```python
from build123d import *

# Parameters (mm, degrees)
SKETCH4_W                = 12.46
SKETCH4_H                = 17.25
BOSS_EXTRUDE3_DEPTH      = 6
SKETCH8_R                = 12.546781182
SKETCH8_R_2              = 11.15
BOSS_EXTRUDE6_DEPTH      = 8.3
BOSS_EXTRUDE6_DEPTH_BACK = 17.25
BOSS_EXTRUDE4_DEPTH      = 17.25
SKETCH6_R                = 0.75
CUT_EXTRUDE1_DEPTH       = 5
CHAMFER1_SIZE            = 0.5
CHAMFER1_SIZE2           = 0.866025404
SKETCH10_W               = 12.46
SKETCH10_H               = 23.7
CUT_EXTRUDE3_DEPTH       = 17.25
BOSS_EXTRUDE7_DEPTH      = 8.3
BOSS_EXTRUDE9_DEPTH      = 10
SKETCH20_R               = 11.15
SKETCH20_R_2             = 7.15
BOSS_EXTRUDE11_DEPTH     = 8.3
SKETCH21_R               = 10.15
SKETCH21_R_2             = 7.15
CUT_EXTRUDE7_DEPTH       = 1.3
SKETCH11_W               = 10
SKETCH11_H               = 2
CUT_EXTRUDE4_DEPTH       = 23.7
CUT_EXTRUDE8_REACH       = 37.55
SKETCH25_W               = 12.46
SKETCH25_H               = 6
BOSS_EXTRUDE10_DEPTH     = 35.55
SKETCH18_W               = 21.5
SKETCH18_H               = 11.438292938
CUT_EXTRUDE5_DEPTH       = 2
SKETCH19_R               = 3.5
CUT_EXTRUDE6_DEPTH       = 43.5
CUT_EXTRUDE6_DEPTH_BACK  = 3
FILLET1_R                = 10
SKETCH22_R               = 6.5
BOSS_EXTRUDE12_DEPTH     = 5
SKETCH23_R               = 6.075
BOSS_EXTRUDE13_DEPTH     = 5
FILLET2_R                = 1
BOSS_EXTRUDE14_DEPTH     = 2
CUT_EXTRUDE9_REACH       = 46.5
SKETCH27_R               = 0.75


with BuildPart() as part:
    # Sketch4 → Boss-Extrude3 (new body)
    with BuildSketch(Plane.XY):
        with Locations((0, -1.35)):
            Rectangle(SKETCH4_W, SKETCH4_H)
    extrude(amount=BOSS_EXTRUDE3_DEPTH)



with BuildPart() as body_2:
    # Sketch8 → Boss-Extrude6 (new body, two sides)
    with BuildSketch(Plane(origin=(0, -9.975, 0), x_dir=(-1, 0, 0), z_dir=(0, -1, 0))) as boss_extrude6_sk:
        with Locations((0, -23.55)):
            Circle(SKETCH8_R)
        with Locations((0, -23.55)):
            Circle(SKETCH8_R_2, mode=Mode.SUBTRACT)
    extrude(amount=BOSS_EXTRUDE6_DEPTH)
    extrude(boss_extrude6_sk.sketch, amount=-BOSS_EXTRUDE6_DEPTH_BACK)


with BuildPart() as part_1:
    add(part.part)

    add(body_2.part)  # Boss-Extrude4 merges body 2
    # Sketch5 → Boss-Extrude4 (add)
    with BuildSketch(Plane(origin=(0, 7.275, 0), x_dir=(1, 0, 0), z_dir=(0, 1, 0))):
        with BuildLine():
            Line((12.546781182, -23.55), (12.546781182, 0))
            Line((12.546781182, 0), (6.23, 0))
            Line((6.23, 0), (6.23, -29.7))
            Line((6.23, -29.7), (-6.23, -29.7))
            Line((-6.23, -29.7), (-6.23, 0))
            Line((-6.23, 0), (-12.546781182, 0))
            Line((-12.546781182, 0), (-12.546781182, -23.55))
            ThreePointArc((-12.546781182, -23.55), (0, -36.096781182), (12.546781182, -23.55))
        make_face()
    extrude(amount=-BOSS_EXTRUDE4_DEPTH)

    # Sketch6 → Cut-Extrude1 (cut)
    with BuildSketch(Plane(origin=(0, 7.275, 0), x_dir=(1, 0, 0), z_dir=(0, 1, 0))):
        with Locations((0, -3.6)):
            Circle(SKETCH6_R)
        with Locations((0, -32.1)):
            Circle(SKETCH6_R)
    extrude(amount=-CUT_EXTRUDE1_DEPTH, mode=Mode.SUBTRACT)

    # Chamfer1
    chamfer1_edges = [part_1.edges().sort_by_distance(p)[0] for p in [
        (-0.75, 7.275, 3.6),
        (-0.75, 7.275, 32.1),
    ]]
    chamfer1_side = [part_1.faces().sort_by_distance(p)[0] for p in [
        (0, 7.275, 35.657160381),
    ]]
    chamfer(chamfer1_edges, length=CHAMFER1_SIZE, length2=CHAMFER1_SIZE2, reference=chamfer1_side[0])

    # Sketch10 → Cut-Extrude3 (cut)
    with BuildSketch(Plane(origin=(0, 7.275, 0), x_dir=(1, 0, 0), z_dir=(0, 1, 0))):
        with Locations((0, -17.85)):
            Rectangle(SKETCH10_W, SKETCH10_H)
    extrude(amount=-CUT_EXTRUDE3_DEPTH, mode=Mode.SUBTRACT)

    # Sketch13 → Boss-Extrude7 (add)
    with BuildSketch(Plane.XZ.offset(18.275)):
        with BuildLine():
            Line((-12.546781182, 23.55), (-12.546781182, 0))
            Line((-12.546781182, 0), (12.546781182, 0))
            Line((12.546781182, 0), (12.546781182, 23.55))
            ThreePointArc((12.546781182, 23.55), (0, 11.003218818), (-12.546781182, 23.55))
        make_face()
    extrude(amount=-BOSS_EXTRUDE7_DEPTH)

    # Sketch15 → Boss-Extrude9 (add)
    with BuildSketch(Plane(origin=(0, 7.275, 0), x_dir=(1, 0, 0), z_dir=(0, 1, 0))):
        with BuildLine():
            Line((-12.546781182, 0), (12.546781182, 0))
            Line((12.546781182, 0), (12.546781182, -23.55))
            ThreePointArc((12.546781182, -23.55), (0, -36.096781182), (-12.546781182, -23.55))
            Line((-12.546781182, -23.55), (-12.546781182, 0))
        make_face()
        with BuildLine():
            Line((-6.23, -0.8), (6.23, -0.8))
            Line((6.23, -0.8), (6.23, -33))
            ThreePointArc((6.23, -33), (5.790660172, -34.060660172), (4.73, -34.5))
            Line((4.73, -34.5), (-4.73, -34.5))
            ThreePointArc((-4.73, -34.5), (-5.790660172, -34.060660172), (-6.23, -33))
            Line((-6.23, -33), (-6.23, -0.8))
        make_face(mode=Mode.SUBTRACT)
    extrude(amount=BOSS_EXTRUDE9_DEPTH)

    # Sketch20 → Boss-Extrude11 (add)
    with BuildSketch(Plane.XZ.offset(18.275)):
        with Locations((0, 23.55)):
            Circle(SKETCH20_R)
        with Locations((0, 23.55)):
            Circle(SKETCH20_R_2, mode=Mode.SUBTRACT)
    extrude(amount=-BOSS_EXTRUDE11_DEPTH)

    # Sketch21 → Cut-Extrude7 (cut)
    with BuildSketch(Plane.XZ.offset(18.275)):
        with Locations((0, 23.55)):
            Circle(SKETCH21_R)
        with Locations((0, 23.55)):
            Circle(SKETCH21_R_2, mode=Mode.SUBTRACT)
    extrude(amount=-CUT_EXTRUDE7_DEPTH, mode=Mode.SUBTRACT)

    # Sketch11 → Cut-Extrude4 (cut)
    with BuildSketch(Plane.XY.offset(29.7)):
        with Locations((0, -10.975)):
            Rectangle(SKETCH11_W, SKETCH11_H)
    extrude(amount=-CUT_EXTRUDE4_DEPTH, mode=Mode.SUBTRACT)

    # Sketch25 → Cut-Extrude8 (cut, up to next)
    with BuildSketch(Plane.XZ.offset(18.275), mode=Mode.PRIVATE) as cut_extrude8_sk1:
        with Locations((0, 9)):
            Rectangle(SKETCH25_W, SKETCH25_H)
    cut_extrude8_tool1 = extrude(cut_extrude8_sk1.sketch, amount=-CUT_EXTRUDE8_REACH, mode=Mode.PRIVATE) & part_1.part
    add(cut_extrude8_tool1.solids().sort_by_distance((0, -18.275, 9))[0], mode=Mode.SUBTRACT)

    # Sketch17 → Boss-Extrude10 (add)
    with BuildSketch(Plane(origin=(0, 17.275, 0), x_dir=(1, 0, 0), z_dir=(0, 1, 0))):
        Polygon((22.25, 26.5), (22.25, 0), (-22.25, 0), (-22.25, 26.5), (-18.25, 26.5), (-18.25, 5), (18.25, 5), (18.25, 26.5), align=None)
    extrude(amount=-BOSS_EXTRUDE10_DEPTH)

    # Sketch18 → Cut-Extrude5 (cut)
    with BuildSketch(Plane.ZY.offset(-18.25)):
        with Locations((-15.75, -0.5)):
            Rectangle(SKETCH18_W, SKETCH18_H)
    extrude(amount=-CUT_EXTRUDE5_DEPTH, mode=Mode.SUBTRACT)

    # Sketch19 → Cut-Extrude6 (cut, two sides)
    with BuildSketch(Plane.ZY.offset(-20.25)) as cut_extrude6_sk:
        with Locations((-20, -0.5)):
            Circle(SKETCH19_R)
    extrude(amount=CUT_EXTRUDE6_DEPTH, mode=Mode.SUBTRACT)
    extrude(cut_extrude6_sk.sketch, amount=-CUT_EXTRUDE6_DEPTH_BACK, mode=Mode.SUBTRACT)

    # Fillet1
    fillet1_edges = [part_1.edges().sort_by_distance(p)[0] for p in [
        (20.25, 17.275, -26.5),
        (-20.25, 17.275, -26.5),
        (-20.25, -18.275, -26.5),
        (20.25, -18.275, -26.5),
    ]]
    fillet(fillet1_edges, radius=FILLET1_R)

    # Sketch22 → Boss-Extrude12 (add)
    with BuildSketch(Plane.ZY.offset(22.25)):
        with Locations((-20, -0.5)):
            Circle(SKETCH22_R)
    extrude(amount=-BOSS_EXTRUDE12_DEPTH)

    # Sketch23 → Boss-Extrude13 (add)
    with BuildSketch(Plane(origin=(-17.25, 0, 0), x_dir=(0, 0, -1), z_dir=(1, 0, 0))):
        with Locations((20, -0.5)):
            Circle(SKETCH23_R)
    extrude(amount=BOSS_EXTRUDE13_DEPTH)

    # Fillet2
    fillet2_edges = [part_1.edges().sort_by_distance(p)[0] for p in [
        (-12.25, -0.5, -13.925),
    ]]
    fillet(fillet2_edges, radius=FILLET2_R)

    # Sketch26 → Boss-Extrude14 (add)
    with BuildSketch(Plane.ZY.offset(-20.25)):
        Polygon((-5, 2), (-20, 2.6585), (-26.5, 2.94385), (-26.5, 5.219146469), (-5, 5.219146469), align=None)
        Polygon((-20, -3.6585), (-5, -3), (-5, -6.219146469), (-26.5, -6.219146469), (-26.5, -3.94385), align=None)
    extrude(amount=BOSS_EXTRUDE14_DEPTH)

    # Sketch27 → Cut-Extrude9 (cut, up to next)
    with BuildSketch(Plane(origin=(22.25, 0, 0), x_dir=(0, 0, -1), z_dir=(1, 0, 0)), mode=Mode.PRIVATE) as cut_extrude9_sk1:
        with Locations((10, -0.5)):
            Circle(SKETCH27_R)
    cut_extrude9_tool1 = extrude(cut_extrude9_sk1.sketch, amount=-CUT_EXTRUDE9_REACH, mode=Mode.PRIVATE) & part_1.part
    add(cut_extrude9_tool1.solids().sort_by_distance((22.25, -0.5, -10))[0], mode=Mode.SUBTRACT)


solid = part_1.part
```
Geometry check sheet. Reference: the model listing, model coordinates, mm. A direction names the side the tool comes from. Coordinates: 2 decimals unless noted, no trailing zeros. Order: outer loops, then holes, each group sorted by start corner. A loop starts at its lowest first (then second) coordinate and runs counter-clockwise, first axis right, second up. Notation, with made-up numbers: M -23.75,-30.75 L 9.25,-30.75 A27 ccw 9.25,-8.75 Z; hole C 17.25,33 d7. An arc over 180 degrees is marked long. Answer as a JSON object with one key per item and string values.
Q1. Cross-section at A-A on x = 0. Give the number of separate pieces and of enclosed holes in the cut face, and give its area (3 significant figures).
Results are:
{"separate pieces": "3", "enclosed holes": "0", "area": "514 mm²"}
Q2. Cross-section at B-B on z = 3.6. Record the cut outline in (x, y) (3 decimals).
Results are:
{"outline": "M -12.547,-18.275 L 12.547,-18.275 L 12.547,17.275 L 6.23,17.275 L 6.23,7.275 L 1.25,7.275 L 0.75,6.409 L 0.75,2.275 L -0.75,2.275 L -0.75,6.409 L -1.25,7.275 L -6.23,7.275 L -6.23,17.275 L -12.547,17.275 Z"}
Q3. Depth check by flat-ended pin: pin 1 Ø0.8 at (x, z) = (-0.5, 32) entering from +Y; pin 2 Ø2 at (x, y) = (8, -0.5) entering from -Z; pin 3 Ø0.5 at (y, z) = (-11.5, 29) entering from -X; pin 4 Ø5 at (x, z) = (17, 14.5) entering from +Y. Enter the tip coordinate at first touch or a pass-through.
Results are:
{"pin 1": "stops at y = 6.69", "pin 2": "stops at z = -5", "pin 3": "stops at x = -11.42", "pin 4": "passes through"}
Q4. Tool access check on faces 1 (the flat face through (0, -5, 6)), 2 (the flat face through (19.264, -3.465, -15.6)), 3 (the flat face through (18.25, -11, -16)), 4 (the flat face through (0, 2.275, 32)). Record the directions out of +Z, -Z, +X, -X, +Y, -Y that give a thin tool (end or side, any length) a straight path to the whole face; none if there is none.
Results are:
{"face 1": "+Y, -Y", "face 2": "-Z", "face 3": "-Z, +Y, -Y", "face 4": "+Y"}
Q5. Release check for a two-part mould opening along Z. For faces 5 (the flat face through (-20, 0, -26.5)), 6 (the flat face through (-12.547, -1, 12)), 7 (the flat face through (-6.23, 3, 17)) record: released by +Z, released by -Z, zero draft, split by the parting line, or undercut.
Results are:
{"face 5": "released by -Z", "face 6": "zero draft", "face 7": "undercut"}
Q6. Scan lines: line 1 (Z direction, x = 0, y = 5.1); line 2 (X direction, y = -2, z = -7); line 3 (X direction, y = 0.5, z = 19.5). Record each from-to range of solid material in increasing order.
Results are:
{"line 1": "z = -5 to 2.85, 4.35 to 6, 29.7 to 31.35, 32.85 to 36.1", "line 2": "x = -22.25 to -18.25, 20.25 to 22.25", "line 3": "x = -12.55 to -6.23, 6.23 to 12.55"}
